Autodesk Inventor part; units mm, degrees
ref_plane "YZ Plane" through (0, 0, 0) normal (1, 0, 0) x (0, 1, 0)
ref_plane "XZ Plane" through (0, 0, 0) normal (0, 1, 0) x (-1, 0, 0)
ref_plane "XY Plane" through (0, 0, 0) normal (0, 0, 1) x (1, 0, 0)
sketch "スケッチ1" plane through (0, 0, 0) normal (0, 0, 1) x (1, 0, 0)
  line L0 (-13.5, 13.5) -> (13.5, 13.5) construction
  line L1 (13.5, 13.5) -> (13.5, -13.5) construction
  line L2 (13.5, -13.5) -> (-13.5, -13.5) construction
  line L3 (-13.5, -13.5) -> (-13.5, 13.5) construction
  circle A0 centre (-13.5, 13.5) radius 1.35
  circle A1 centre (13.5, 13.5) radius 1.35
  circle A2 centre (-13.5, -13.5) radius 1.35
  circle A3 centre (13.5, -13.5) radius 1.35
  circle A4 centre (0, 14.5) radius 10.5 construction
  line L4 (-6.25, -25) -> (6.25, -25) construction
  line L5 (6.25, -25) -> (6.25, -30) construction
  line L6 (6.25, -30) -> (-6.25, -30) construction
  line L7 (-6.25, -30) -> (-6.25, -25) construction
  line L8 (-16.25, -25) -> (16.25, -25) construction
  line L9 (16.25, -25) -> (16.25, -30) construction
  line L10 (16.25, -30) -> (-16.25, -30) construction
  line L11 (-16.25, -30) -> (-16.25, -25) construction
  line L12 (-6.3, -24.95) -> (6.3, -24.95) construction
  line L13 (6.3, -24.95) -> (6.3, -30.05) construction
  line L14 (6.3, -30.05) -> (-6.3, -30.05) construction
  line L15 (-6.3, -30.05) -> (-6.3, -24.95) construction
  circle A5 centre (-5.25, -24.95) radius 1.05 construction
  circle A6 centre (-11.25, -27.5) radius 1.55
  circle A7 centre (11.25, -27.5) radius 1.55
  line L16 (0, 0) -> (0, -13.5) construction
  line L17 (-6.3, -24.95) -> (-6.3, -30.05)
  line L18 (6.3, -27.5) -> (-6.3, -27.5) construction
  line L19 (0, -25) -> (0, -30.05) construction
  arc A8 (-4.2, -24.95) -> (-6.3, -24.95) centre (-5.25, -24.95) ccw
  arc A9 (-6.3, -30.05) -> (-4.2, -30.05) centre (-5.25, -30.05) ccw
  line L20 (-4.2, -24.95) -> (4.2, -24.95)
  line L21 (-4.2, -30.05) -> (4.2, -30.05)
  arc A10 (6.3, -24.95) -> (4.2, -24.95) centre (5.25, -24.95) ccw
  arc A11 (4.2, -30.05) -> (6.3, -30.05) centre (5.25, -30.05) ccw
  line L22 (6.3, -24.95) -> (6.3, -30.05)
  circle A12 centre (-13.5, -13.5) radius 2.75 construction
  circle A13 centre (13.5, 13.5) radius 2.75 construction
  line L23 (-16.25, -13.5) -> (-16.25, -30)
  line L24 (-16.25, -30) -> (-6.25, -33)
  line L25 (-6.25, -33) -> (6.25, -33)
  line L26 (6.25, -33) -> (16.25, -30)
  line L27 (16.25, -30) -> (16.25, 13.5)
  arc A14 (16.25, 13.5) -> (10.7575, 13.7031) centre (13.5, 13.5) ccw
  arc A15 (6.7066, 6.0513) -> (10.7575, 13.7031) centre (0, 14.5) ccw
  line L28 (6.7066, 6.0513) -> (-15.2098, -11.3461)
  arc A16 (-15.2098, -11.3461) -> (-16.25, -13.5) centre (-13.5, -13.5) ccw
  line L29 (-10.75, -14.1897) -> (-10.75, -22)
  line L30 (-10.75, -22) -> (10.75, -22)
  line L31 (10.75, -22) -> (10.75, 2.8772)
  line L32 (10.75, 2.8772) -> (-10.75, -14.1897)
  point P0 (0, 13.5)
  point P1 (13.5, 0)
  point P2 (-16.25, -27.5)
  dimension "d23" = 2.1
  dimension "d0" = 27
  dimension "d3" = 27
  dimension "d6" = 27
  dimension "d9" = 2.7
  dimension "d10" = 21
  dimension "d11" = 1
  dimension "d12" = 11.5
  dimension "d13" = 5
  dimension "d16" = 32.5
  dimension "d20" = 10
  dimension "d22" = 0.05
  dimension "d24" = 5
  dimension "d26" = 3.1
  dimension "d31" = 5.5
  dimension "d32" = 3
  dimension "d33" = 5
  dimension "d34" = 3
extrude "押し出し1" add sketch "スケッチ1" along normal blind 2 contours A16 L28 A15 A14 L27 L26 L25 L24 L23 | L32 L31 L30 L29
fillet "フィレット1" radius 4 4 edges at (16.25, -30, 1) (-16.25, -30, 1) (-6.25, -33, 1) (6.25, -33, 1)
sketch "スケッチ2" plane through (0, 0, 2) normal (0, 0, 1) x (1, 0, 0)
  circle A0 centre (-13.5, -13.5) radius 1.35
  circle A1 centre (-13.5, -13.5) radius 1.35
  circle A2 centre (13.5, -13.5) radius 1.35
  circle A3 centre (13.5, -13.5) radius 1.35
  circle A4 centre (11.25, -27.5) radius 1.55
  circle A5 centre (11.25, -27.5) radius 1.55
  circle A6 centre (-11.25, -27.5) radius 1.55
  circle A7 centre (-11.25, -27.5) radius 1.55
  circle A8 centre (13.5, 13.5) radius 1.35
  circle A9 centre (13.5, 13.5) radius 1.35
  point P0 (0, 0)
extrude "押し出し2" add sketch "スケッチ2" against normal up to surface (2 mm away)
equation "\"d3\" = d0"
equation "\"d6\" = d0"
equation "\"d16\" = d0_1"
equation "\"d20\" = d3_1"
equation "\"d24\" = d17"
equation "\"d34\" = d32"
properties part number "上腕_サブフレーム_1_1" material "GFRP"
Could you check a few things on this model? Use its own coordinates, in mm. A direction names the side the tool comes from. Give positions to 0.01 mm unless a question says otherwise; leave off trailing zeros. Order: outer loops, then holes, each group sorted by start corner. A loop starts at its lowest first (then second) coordinate and runs counter-clockwise, first axis right, second up. Notation, with made-up numbers: (39, 3) - (52, 3) arc R25 ccw to (52, 33) - close; hole circle Ø4 at (84.5, -5). An arc over 180 degrees is marked (long way). Return JSON: item names as keys, results as strings. Group by question number.
Q1. Please list where these lines run through material, in increasing order: line 1 along X through (y, z) = (-26, 0.1); line 2 along Y through (x, z) = (-3, 1.3); line 3 along Y through (x, z) = (-1, 0.4). Write a range as [from, to].
Q2. Suppose I cut it at A-A, the plane y = -26. Please give me the cut outline in (x, z).
Q3. Suppose I cut it at D-D, the plane x = -9. Please give me the cut outline in (y, z) (3 decimals), and give its area (3 significant figures).
Q4. Which directions (+Z, -Z, +X, -X, +Y, -Y) give clear straight access to the entire face, cutting with the end or side of a thin tool? Please do faces 1 (the face through (6.3, -27, 1)), 2 (the face through (16.25, -7, 1)).
Q5. Suppose I cut it at C-C, the plane x = -2.5. Please give me the cut outline in (y, z).
Q6. Thinking about a two-plate mould opening in X: for faces 3 (the face through (10.06, -31.857, 0.986)), 4 (the face through (0, -30.05, 1)), 5 (the face through (-15.48, -29.38, 1.01)), 6 (the face through (0, -24.95, 1)), which applies, pulls with the +X half, pulls with the -X half, needs draft (parallel to the pull), parting line crosses it, or undercut?
Q7. Suppose I cut it at B-B, the plane z = 1.05. Please give me the cut outline in (x, y).
Resolved:
{
 "1": {"line 1": "x = [-16.25, -6.3], [6.3, 16.25]", "line 2": "y = [-33, -30.05], [-24.95, -1.65]", "line 3": "y = [-33, -30.05], [-24.95, -0.07]"},
 "2": {"outline": "(-16.25, 0) - (-6.3, 0) - (-6.3, 2) - (-16.25, 2) - close; (6.3, 0) - (16.25, 0) - (16.25, 2) - (6.3, 2) - close"},
 "3": {"outline": "(-32.175, 0) - (-6.417, 0) - (-6.417, 2) - (-32.175, 2) - close", "area": "51.5 mm2"},
 "4": {"face 1": "+Z, -Z", "face 2": "+Z, -Z, +X, +Y, -Y"},
 "5": {"outline": "(-33, 0) - (-30.05, 0) - (-30.05, 2) - (-33, 2) - close; (-24.95, 0) - (-1.26, 0) - (-1.26, 2) - (-24.95, 2) - close"},
 "6": {"face 3": "pulls with the +X half", "face 4": "undercut", "face 5": "pulls with the -X half", "face 6": "undercut"},
 "7": {"outline": "(-16.25, -27.02) arc R4 ccw to (-13.4, -30.86) - (-6.81, -32.83) arc R4 ccw to (-5.66, -33) - (5.66, -33) arc R4 ccw to (6.81, -32.83) - (13.4, -30.86) arc R4 ccw to (16.25, -27.02) - (16.25, 13.5) arc R2.75 ccw to (10.76, 13.7) arc R10.79 cw to (6.71, 6.05) - (-15.21, -11.35) arc R2.75 ccw to (-16.25, -13.5) - close; hole (-6.3, -30.05) arc R1.05 ccw to (-4.2, -30.05) - (4.2, -30.05) arc R1.05 ccw to (6.3, -30.05) - (6.3, -24.95) arc R1.05 ccw to (4.2, -24.95) - (-4.2, -24.95) arc R1.05 ccw to (-6.3, -24.95) - close"}
}
